For this review, use the dimensioned drawing (mm, ordinates from the lowest corner) and the shaded views. Coordinates: 2 decimals unless noted, no trailing zeros. Loops run counter-clockwise (first coordinate to the right, second up) from the corner with the lowest first, then second, coordinate; pieces in that order, holes last. Notation, with made-up numbers: M -0.75,28 L 30.25,28 A25 cw 30.25,62 Z; hole C 39.5,65.25 d6. An arc over 180 degrees is marked long. Write item = value, one per line. Start each with the question number.
Q1. We need section C-C on x = 24. Give the boundary of the cut face in (y, z) (1 decimal), and give its area (3 significant figures).
Q2. We need section B-B on y = 31. Give the boundary of the cut face in (x, z) (1 decimal), and give its area (3 significant figures).
Q3. We need section A-A on z = 7.25. Give the boundary of the cut face in (x, y), and give its area (3 significant figures).
Q4. Clearance check with flat-ended pins moving along their axes: pin 1 Ø8 at (x, z) = (33, 2) entering from +Y; pin 2 Ø1 at (x, z) = (34.5, 6) entering from +Y (1 decimal); pin 3 Ø5.5 at (x, z) = (20.61, 7.41) entering from +Y. State where each tip first meets the part, or that it passes through.
Q5. Wall thickness on probe 1 along Z at (x, y) = (20.5, 37) (1 decimal); probe 2 along X at (y, z) = (30, 13.75) (1 decimal); probe 3 along X at (y, z) = (22.5, 4.25): over which ranges is each line inside the solid? List them lowest first.
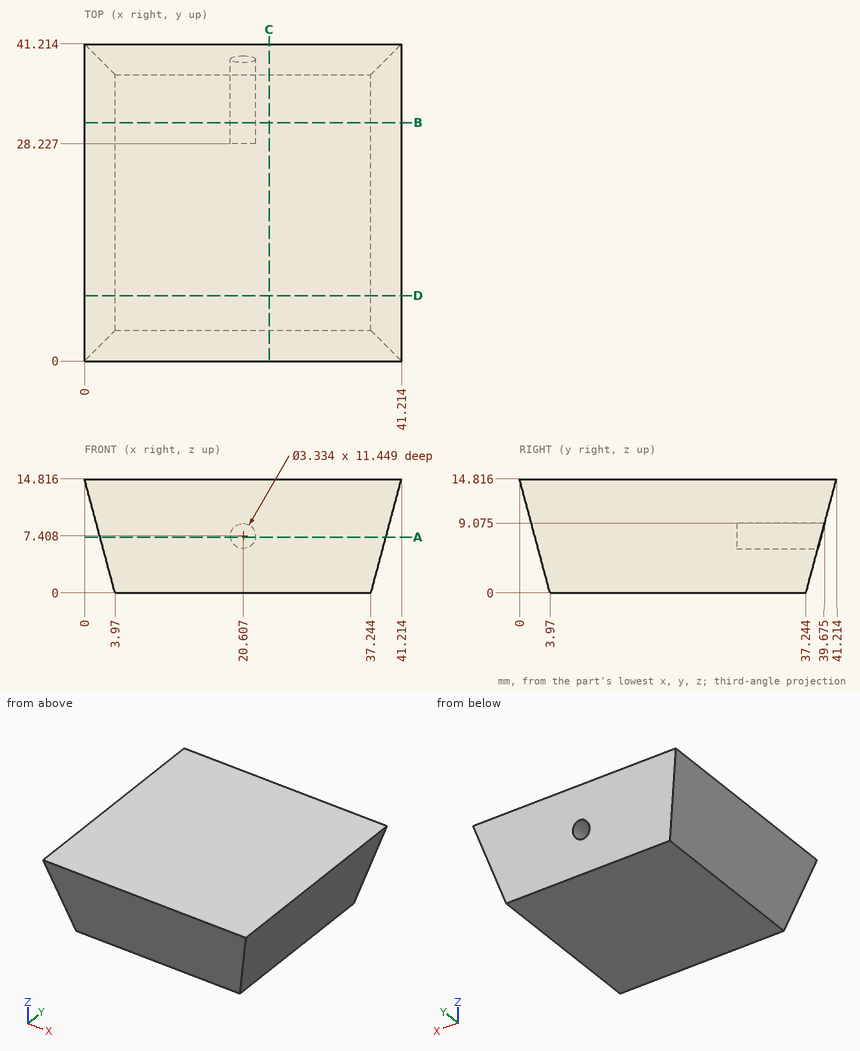
Returned:
q1.outline = M 0,14.8 L 4,0 L 37.2,0 L 41.2,14.8 Z
q1.area = 552 mm^2
q2.outline = M 0,14.8 L 4,0 L 37.2,0 L 41.2,14.8 Z; hole C 20.6,7.4 d3.3
q2.area = 543 mm^2
q3.outline = M 2.03,2.03 L 39.19,2.03 L 39.19,39.19 L 22.27,39.19 L 22.27,28.23 L 18.95,28.23 L 18.95,39.19 L 2.03,39.19 Z
q3.area = 1,340 mm^2
q4.pin_1 = 38.85
q4.pin_2 = 39
q4.pin_3 = 39.97
q5.probe_1 = 0 to 5.7, 9.1 to 14.8
q5.probe_2 = 0.3 to 40.9
q5.probe_3 = 2.83 to 38.38
